Could you check a few things on this model? Use its own coordinates, in mm. Face numbers are marked on the shaded views. A direction names the side the tool comes from. Round coordinates to 2 decimals unless told otherwise and drop trailing zeros. Loops run counter-clockwise (first coordinate to the right, second up) from the corner with the lowest first, then second, coordinate; pieces in that order, holes last. Notation, with made-up numbers: (-1.5, 2.5) - (7.5, 2.5) arc R22 ccw to (7.5, 24.5) - close; hole circle Ø8 at (-15.5, 7.25). An arc over 180 degrees is marked (long way). Use one line per item in the form item = value.
```python
from build123d import *

# Parameters (mm, degrees)
CROQUIS2_R              = 12.7
CROQUIS2_R_2            = 9.525
SALIENTE_EXTRUIR1_DEPTH = 51.435
CORTAR_EXTRUIR1_START   = -5.08
CROQUIS3_R              = 12.7
CORTAR_EXTRUIR1_DEPTH   = 71.699448436
CROQUIS4_R              = 3.33375
SALIENTE_EXTRUIR3_DEPTH = 6.35
CROQUIS4_2_R            = 3.33375
CORTAR_EXTRUIR3_DEPTH   = 76.779448436
REDONDEO3_R             = 2.54


with BuildPart() as part:
    # Croquis2 → Saliente-Extruir1 (new body)
    # profile 1 of 2: a face of its own
    with BuildSketch(Plane(origin=(0, 0, 0), x_dir=(1, 0, 0), z_dir=(0, 1, 0))):
        with BuildLine():
            Line((41.7195, 6.35), (11.662827783, 32.470389268))
            ThreePointArc((11.662827783, 32.470389268), (6.225507161, 35.70447269), (0, 36.83))
            ThreePointArc((0, 36.83), (-6.225507161, 35.70447269), (-11.662827783, 32.470389268))
            Line((-11.662827783, 32.470389268), (-41.7195, 6.35))
            Line((-41.7195, 6.35), (-41.7195, 0))
            Line((-41.7195, 0), (41.7195, 0))
            Line((41.7195, 0), (41.7195, 6.35))
        make_face()
        with Locations((0, 19.05)):
            Circle(CROQUIS2_R, mode=Mode.SUBTRACT)
    # profile 2 of 2: a face of its own
    with BuildSketch(Plane(origin=(0, 0, 0), x_dir=(1, 0, 0), z_dir=(0, 1, 0))):
        with Locations((0, 19.05)):
            Circle(CROQUIS2_R)
        with Locations(Location((0, 19.05, 0), (0, 0, 270))):
            Circle(CROQUIS2_R_2, mode=Mode.SUBTRACT)
    extrude(amount=-SALIENTE_EXTRUIR1_DEPTH)

    # Croquis3 → Cortar-Extruir1 (cut, through all)
    with BuildSketch(Plane(origin=(0, 0, 0), x_dir=(1, 0, 0), z_dir=(0, 1, 0)).offset(CORTAR_EXTRUIR1_START)):
        with Locations(Location((0, 19.05, 0), (0, 0, 270))):
            Circle(CROQUIS3_R)
    extrude(amount=-CORTAR_EXTRUIR1_DEPTH, mode=Mode.SUBTRACT)

    # Croquis4 → Saliente-Extruir3 (add)
    with BuildSketch(Plane.XY):
        with Locations((-36.000000009, -5.717499995)):
            Circle(CROQUIS4_R)
        with Locations((36.000000009, -5.717499995)):
            Circle(CROQUIS4_R)
        with Locations((36.000000009, -45.717500005)):
            Circle(CROQUIS4_R)
        with Locations((-36.000000009, -45.717500005)):
            Circle(CROQUIS4_R)
    extrude(amount=-SALIENTE_EXTRUIR3_DEPTH)

    # Croquis4<2> → Cortar-Extruir3 (cut, through all)
    with BuildSketch(Plane.XY):
        with Locations((-36.000000009, -5.717499995)):
            Circle(CROQUIS4_2_R)
        with Locations((36.000000009, -5.717499995)):
            Circle(CROQUIS4_2_R)
        with Locations((36.000000009, -45.717500005)):
            Circle(CROQUIS4_2_R)
        with Locations((-36.000000009, -45.717500005)):
            Circle(CROQUIS4_2_R)
    extrude(amount=-CORTAR_EXTRUIR3_DEPTH, mode=Mode.SUBTRACT)

    # Redondeo3
    # the kernel refuses this fillet: 2.54 mm, written as the material it takes off along each edge
    with BuildSketch(Plane(origin=(41.7195, 2.894405132, -6.35), x_dir=(-0.7548025459958689, 0, -0.6559520687963062), z_dir=(0, -1, 0))) as redondeo3_piece_1:
        with BuildLine():
            CenterArc((REDONDEO3_R * 0.455811831887, -REDONDEO3_R), REDONDEO3_R, 90, 49.008119667)
            Line((-REDONDEO3_R * 0.298990714108, -REDONDEO3_R * 0.344047931204), (0, 0))
            Line((0, 0), (REDONDEO3_R * 0.455811831887, 0))
        make_face()
    extrude(amount=57.223810265, mode=Mode.SUBTRACT)
    with BuildSketch(Plane(origin=(41.7195, 6.35, 0), x_dir=(0, 0, -1), z_dir=(0, -1, 0)), Plane(origin=(-41.7195, 6.35, 0), x_dir=(1, 0, 0), z_dir=(0, -1, 0))) as redondeo3_piece_2:
        with BuildLine():
            CenterArc((REDONDEO3_R, -REDONDEO3_R), REDONDEO3_R, 90, 90)
            Line((0, -REDONDEO3_R), (0, 0))
            Line((0, 0), (REDONDEO3_R, 0))
        make_face()
    extrude(amount=64.135, mode=Mode.SUBTRACT)
    with BuildSketch(Plane(origin=(-41.7195, 2.894405132, -6.35), x_dir=(0.7548025459958687, 0, -0.6559520687963067), z_dir=(0, -1, 0))) as redondeo3_piece_3:
        with BuildLine():
            CenterArc((REDONDEO3_R * 0.455811831887, REDONDEO3_R), REDONDEO3_R, 220.991880333, 49.008119667)
            Line((-REDONDEO3_R * 0.298990714108, REDONDEO3_R * 0.344047931204), (0, 0))
            Line((0, 0), (REDONDEO3_R * 0.455811831887, 0))
        make_face()
    extrude(amount=57.223810265, mode=Mode.SUBTRACT)


solid = part.part
```
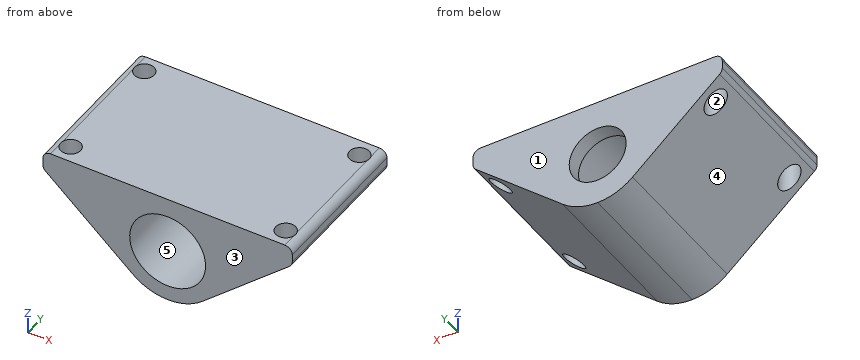
1. If we section it at D-D, the plane x = -3: Write out the boundary of the cut face in (y, z) (3 decimals), plus the area to 3 significant figures.
Solution:
outline = (-51.435, -36.575) - (0, -36.575) - (0, -28.09) - (-5.08, -28.09) - (-5.08, -31.391) - (-51.435, -31.391) - close; (-51.435, -6.709) - (-5.08, -6.709) - (-5.08, -10.01) - (0, -10.01) - (0, 0) - (-51.435, 0) - close
area = 645 mm^2
2. Please list where these lines run through material, in increasing order: line 1 along Y through (x, z) = (-36, -10) (3 decimals); line 2 along X through (y, z) = (-16.5, -30); line 3 along X through (y, z) = (-36, -23.5).
Solution:
line_1 = -51.435 to -49.051, -42.384 to -9.051, -2.384 to 0
line_2 = -14.51 to -6.43, 6.43 to 14.51
line_3 = -21.99 to -11.89, 11.89 to 21.99
3. If we section it at A-A, the plane y = -38: Write out the boundary of the cut face in (x, z).
Solution:
outline = (-41.72, -5.19) arc R2.54 ccw to (-40.85, -7.11) - (-11.66, -32.47) arc R17.78 ccw to (11.66, -32.47) - (40.85, -7.11) arc R2.54 ccw to (41.72, -5.19) - (41.72, -2.54) arc R2.54 ccw to (39.18, 0) - (-39.18, 0) arc R2.54 ccw to (-41.72, -2.54) - close; hole circle Ø25.4 at (0, -19.05)
4. We'd pull the mould along Y, two halves only. Please class the marked faces 1, 2 and 3: +Y half, -Y half, draft (parallel to the pull), parting line (faces both ways), or undercut.
Solution:
face_1 = +Y half
face_2 = undercut
face_3 = -Y half
5. For P1, Ø5, axis at x = 17.5, y = -41, coming from the -Z side; P2, Ø5, axis at y = -42.5, z = -27.5, coming from the +X side; P3, Ø8.5, axis at x = 36, y = -45.72, coming from the -Z side, each with a flat end and sliding along its axis, tell me the tip position at first contact or that it passes through.
Solution:
P1 = -29.57
P2 = 20.26
P3 = -15.01
6. If we section it at B-B, the plane z = -11: Write out the boundary of the cut face in (x, y) (1 decimal), plus the area to 3 significant figures.
Solution:
outline = (-36.4, -51.4) - (-9.8, -51.4) - (-9.8, -5.1) - (-5.1, -5.1) - (-5.1, 0) - (-36.4, 0) - (-36.4, -2.4) arc R3.3 cw (long way) to (-36.4, -9) - (-36.4, -42.4) arc R3.3 cw (long way) to (-36.4, -49) - close; (5.1, -5.1) - (9.8, -5.1) - (9.8, -51.4) - (36.4, -51.4) - (36.4, -49) arc R3.3 cw (long way) to (36.4, -42.4) - (36.4, -9) arc R3.3 cw (long way) to (36.4, -2.4) - (36.4, 0) - (5.1, 0) - close
area = 2,700 mm^2
7. If we section it at C-C, the plane x = -36: Write out the boundary of the cut face in (y, z) (3 decimals), plus the area to 3 significant figures.
Solution:
outline = (-51.435, -11.32) - (-49.051, -11.32) - (-49.051, 0) - (-51.435, 0) - close; (-42.384, -11.32) - (-9.051, -11.32) - (-9.051, 0) - (-42.384, 0) - close; (-2.384, -11.32) - (0, -11.32) - (0, 0) - (-2.384, 0) - close
area = 431 mm^2
8. On a 3-axis mill with a long thin cutter (end or side, diameter ignored), from which of +Z, -Z, +X, -X, +Y, -Y can I reach the whole of each face in a straight line? I mean the marked faces 4 and 5. Say none if no direction works.
Solution:
face_4 = -Z, -X, +Y, -Y
face_5 = -Y
